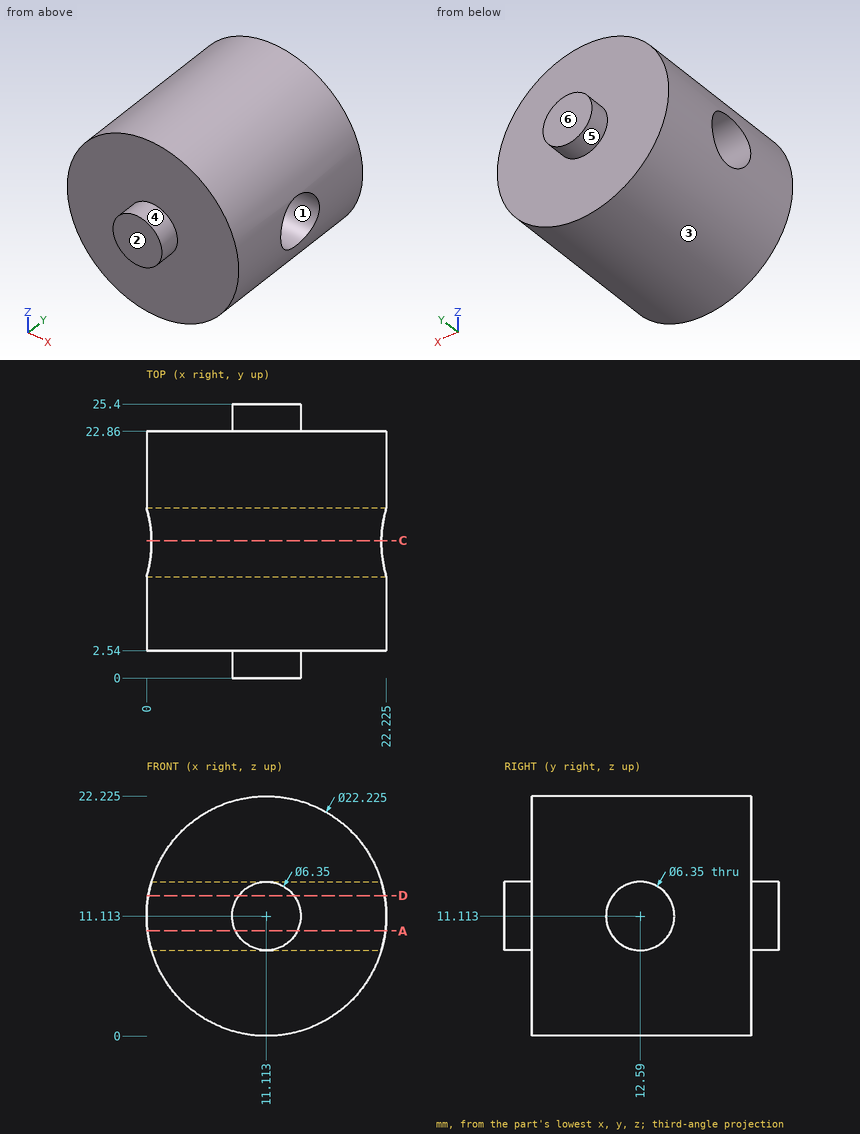
Could you check a few things on this drawing? It's one solid part, dimensions in mm from its lowest x, y, z. A direction names the side the tool comes from. Coordinates: 2 decimals unless noted, no trailing zeros. Order: outer loops, then holes, each group sorted by start corner. A loop starts at its lowest first (then second) coordinate and runs counter-clockwise, first axis right, second up. Notation, with made-up numbers: (31, 27) - (57, 27) arc R19 cw to (57, 44) - close; hole circle Ø7 at (45, -10). An arc over 180 degrees is marked (long way). Answer as a JSON object with one key per item and string values. Group by question number.
Q1. Imagine slicing it at C-C (y = 12.75). Please give me the cut outline in (x, z) (1 decimal), and give its area (3 significant figures).
Q2. Imagine slicing it at D-D (z = 13). Please give me the cut outline in (x, y) (1 decimal).
Q3. Imagine slicing it at A-A (z = 9.75). Please give me the cut outline in (x, y) (1 decimal).
Q4. I need wall thicknesses on line 1 (Y direction, x = 11, z = 6.75); line 2 (Y direction, x = 19.5, z = 13.5) (1 decimal); line 3 (Y direction, x = 2.25, z = 8.25) (1 decimal). Which ranges of each line are inside material? Lowest first, please. Write a range as from..to.
Q5. On a 3-axis mill with a long thin cutter (end or side, diameter ignored), from which of +Z, -Z, +X, -X, +Y, -Y can I reach the whole of each face in a straight line? I mean the marked faces 4, 5 and 6. Say none if no direction works.
Q6. Will these pins go through, and if not, where does the flat tip stop? P1, Ø1, axis at x = 13.5, z = 14, coming from the +Y side; P2, Ø1.5, axis at y = 6.5, z = 15, coming from the +X side; P3, Ø1.5, axis at y = 12.5, z = 19.5, coming from the +X side (1 decimal); P4, Ø10, axis at x = 10, z = 18, coming from the +Y side.
Q7. We'd pull the mould along Z, two halves only. Please class the marked faces 1, 2 and 3: +Z half, -Z half, draft (parallel to the pull), parting line (faces both ways), or undercut.
Determined:
{
 "1": {"outline": "(0.5, 7.9) arc R11.1 ccw to (21.8, 7.9) - close; (0.5, 14.3) - (21.8, 14.3) arc R11.1 ccw to start", "area": "249 mm2"},
 "2": {"outline": "(0.2, 2.5) - (8.6, 2.5) - (8.6, 0) - (13.7, 0) - (13.7, 2.5) - (22.1, 2.5) - (22.1, 10) - (0.2, 10) - close; (0.2, 15.1) - (22.1, 15.1) - (22.1, 22.9) - (13.7, 22.9) - (13.7, 25.4) - (8.6, 25.4) - (8.6, 22.9) - (0.2, 22.9) - close"},
 "3": {"outline": "(0.1, 2.5) - (8.2, 2.5) - (8.2, 0) - (14, 0) - (14, 2.5) - (22.1, 2.5) - (22.1, 9.7) - (0.1, 9.7) - close; (0.1, 15.5) - (22.1, 15.5) - (22.1, 22.9) - (14, 22.9) - (14, 25.4) - (8.2, 25.4) - (8.2, 22.9) - (0.1, 22.9) - close"},
 "4": {"line 1": "y = 2.54..22.86", "line 2": "y = 2.5..10.5, 14.7..22.9", "line 3": "y = 2.5..11.2, 14..22.9"},
 "5": {"face 4": "-Y", "face 5": "+Y", "face 6": "+Z, -Z, +X, -X, +Y"},
 "6": {"P1": "stops at y = 22.86", "P2": "stops at x = 21.77", "P3": "stops at x = 19.2", "P4": "stops at y = 25.4"},
 "7": {"face 1": "undercut", "face 2": "draft", "face 3": "parting line"}
}
